```python
from build123d import *
from build123d import SkipClean  # not in build123d's __all__

# Parameters (mm, degrees)
F0_R      = 7.925
F1_DEPTH  = 9.6
F2_R      = 6.425
F3_DEPTH  = 2.5
F4_R      = 2.3
F4_R_2    = 1.575
F5_DEPTH  = 1.82
F12_W     = 4
F12_H     = 4.34
F13_DEPTH = 22.4162849636
F10_W     = 4
F10_H     = 4.34
F14_DEPTH = 22.4162849636
F17_DEPTH = 9.6
F15_R     = 2.4
F18_DEPTH = 15.851


with BuildPart() as f1:
    # F0 (on Top) → F1 (new body)
    with BuildSketch(Plane.XY):
        Circle(F0_R)
    extrude(amount=F1_DEPTH)

    # F2 (on face) → F3 (cut)
    with BuildSketch(Plane(origin=(0, 0, 0), x_dir=(1, 0, 0), z_dir=(0, 0, -1))):
        Circle(F2_R)
    extrude(amount=-F3_DEPTH, mode=Mode.SUBTRACT)

    # F4 (on face) → F5 (join)
    with BuildSketch(Plane.XY.offset(9.6)):
        with Locations((-4.1473636204, -3.8)):
            Circle(F4_R)
        with Locations((-4.1473636204, -3.8)):
            Circle(F4_R_2, mode=Mode.SUBTRACT)
        with Locations((-4.1473636204, 3.8)):
            Circle(F4_R)
        with Locations((-4.1473636204, 3.8)):
            Circle(F4_R_2, mode=Mode.SUBTRACT)
        with Locations((4.1473636204, 3.8)):
            Circle(F4_R)
        with Locations((4.1473636204, 3.8)):
            Circle(F4_R_2, mode=Mode.SUBTRACT)
        with Locations((4.1473636204, -3.8)):
            Circle(F4_R)
        with Locations((4.1473636204, -3.8)):
            Circle(F4_R_2, mode=Mode.SUBTRACT)
    extrude(amount=F5_DEPTH)

    # F12 (on face) → F13 (cut, through all)
    with BuildSketch(Plane(origin=(7.925, 7.925, 0), x_dir=(-0.7071067812, 0.7071067812, 0), z_dir=(0.7071067812, 0.7071067812, 0))):
        Rectangle(F12_W, F12_H)
    extrude(amount=-F13_DEPTH, mode=Mode.SUBTRACT)

    # F10 (on face) → F14 (cut, through all)
    with BuildSketch(Plane(origin=(7.925, -7.925, 0), x_dir=(0.7071067812, 0.7071067812, 0), z_dir=(0.7071067812, -0.7071067812, 0))):
        Rectangle(F10_W, F10_H)
    extrude(amount=-F14_DEPTH, mode=Mode.SUBTRACT)

    # F16 (on face) → F17 (join)
    with BuildSketch(Plane.XY.offset(9.6)):
        with BuildLine():
            Line((1.6, 2.828869032), (1.6, 3.5))
            Line((1.6, 3.5), (-1.6, 3.5))
            Line((-1.6, 3.5), (-1.6, 2.828869032))
            ThreePointArc((-1.6, 2.828869032), (-1.4275666191, 2.9196838096), (-1.25, 3))
            ThreePointArc((-1.25, 3), (0, 3.25), (1.25, 3))
            ThreePointArc((1.25, 3), (1.4275666191, 2.9196838096), (1.6, 2.828869032))
        make_face()
        with BuildLine():
            ThreePointArc((3.25, 0), (2.8073564077, 1.6374522894), (1.6, 2.828869032))
            Line((1.6, 2.828869032), (1.6, 1.9209372712))
            ThreePointArc((1.6, 1.9209372712), (2.2638462845, 1.0606601718), (2.5, 0))
            ThreePointArc((2.5, 0), (2.2638462845, -1.0606601718), (1.6, -1.9209372712))
            Line((1.6, -1.9209372712), (1.6, -2.828869032))
            ThreePointArc((1.6, -2.828869032), (2.8073564077, -1.6374522894), (3.25, 0))
        make_face()
        with BuildLine():
            Line((1.6, 1.9209372712), (1.6, 2.828869032))
            ThreePointArc((1.6, 2.828869032), (1.4275666191, 2.9196838096), (1.25, 3))
            Line((1.25, 3), (1.25, 2.1650635095))
            ThreePointArc((1.25, 2.1650635095), (1.4302183068, 2.0504817958), (1.6, 1.9209372712))
        make_face()
        with BuildLine():
            ThreePointArc((-1.25, 3), (-1.4275666191, 2.9196838096), (-1.6, 2.828869032))
            Line((-1.6, 2.828869032), (-1.6, 1.9209372712))
            ThreePointArc((-1.6, 1.9209372712), (-1.4302183068, 2.0504817958), (-1.25, 2.1650635095))
            Line((-1.25, 2.1650635095), (-1.25, 3))
        make_face()
        with BuildLine():
            Line((-1.6, 1.9209372712), (-1.6, 2.828869032))
            ThreePointArc((-1.6, 2.828869032), (-3.25, 0), (-1.6, -2.828869032))
            Line((-1.6, -2.828869032), (-1.6, -1.9209372712))
            ThreePointArc((-1.6, -1.9209372712), (-2.5, 0), (-1.6, 1.9209372712))
        make_face()
        with BuildLine():
            ThreePointArc((-1.25, -3), (-1.4275666191, -2.9196838096), (-1.6, -2.828869032))
            Line((-1.6, -2.828869032), (-1.6, -3.5))
            Line((-1.6, -3.5), (1.6, -3.5))
            Line((1.6, -3.5), (1.6, -2.828869032))
            ThreePointArc((1.6, -2.828869032), (1.4275666191, -2.9196838096), (1.25, -3))
            ThreePointArc((1.25, -3), (0, -3.25), (-1.25, -3))
        make_face()
        with BuildLine():
            Line((-1.6, -1.9209372712), (-1.6, -2.828869032))
            ThreePointArc((-1.6, -2.828869032), (-1.4275666191, -2.9196838096), (-1.25, -3))
            Line((-1.25, -3), (-1.25, -2.1650635095))
            ThreePointArc((-1.25, -2.1650635095), (-1.4302183068, -2.0504817958), (-1.6, -1.9209372712))
        make_face()
        with BuildLine():
            Line((1.6, -2.828869032), (1.6, -1.9209372712))
            ThreePointArc((1.6, -1.9209372712), (1.4302183068, -2.0504817958), (1.25, -2.1650635095))
            Line((1.25, -2.1650635095), (1.25, -3))
            ThreePointArc((1.25, -3), (1.4275666191, -2.9196838096), (1.6, -2.828869032))
        make_face()
        with BuildLine():
            Line((-1.25, 3), (1.25, 3))
            ThreePointArc((1.25, 3), (0, 3.25), (-1.25, 3))
        make_face()
        with BuildLine():
            Line((1.25, -3), (-1.25, -3))
            ThreePointArc((-1.25, -3), (0, -3.25), (1.25, -3))
        make_face()
    with SkipClean():  # cleaning this boolean's faces spoils the solid; the shape is the same uncleaned
        extrude(amount=-F17_DEPTH)

    # F15 (on offset) → F18 (cut, through all)
    with BuildSketch(Plane.YZ.offset(7.925)):
        with Locations((0, 5.4)):
            Circle(F15_R)
    with SkipClean():  # cleaning this boolean's faces spoils the solid; the shape is the same uncleaned
        extrude(amount=-F18_DEPTH, mode=Mode.SUBTRACT)


solid = f1.part
```
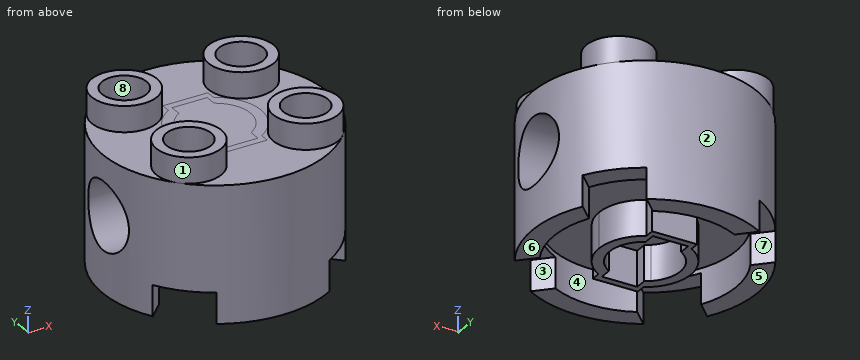
The listing builds one solid part. Answer for the finished solid, in the listing's coordinates (mm). Face numbers are marked on the shaded views. A direction names the side the tool comes from. Round coordinates to 2 decimals unless told otherwise and drop trailing zeros. Write each loop counter-clockwise with the first axis right and the second up, starting at its lowest first coordinate (ties: lowest second). Pieces come first, ordered by that corner, then holes. Notation, with made-up numbers: (14, -38.75) -> (57, -38.75) arc R21 cw to (57, -22.75) -> close; hole circle Ø1 at (-24.5, 21.25). An arc over 180 degrees is marked (long way). Write item = value, one per line.
1) Section B-B on y = 0.75 is taken. Write down the section's boundary in (x, z).
Check values:
outline = (-7.89, 0) -> (-6.38, 0) -> (-6.38, 2.5) -> (-3.16, 2.5) -> (-3.16, 0) -> (-2.38, 0) -> (-2.38, 2.5) -> (2.38, 2.5) -> (2.38, 0) -> (3.16, 0) -> (3.16, 2.5) -> (6.38, 2.5) -> (6.38, 0) -> (7.89, 0) -> (7.89, 3.12) -> (-7.89, 3.12) -> close; (-7.89, 7.68) -> (7.89, 7.68) -> (7.89, 9.6) -> (-7.89, 9.6) -> close
2) Straight lines are drawn through the part: line 1 along X through (y, z) = (-4.25, 10); line 2 along X through (y, z) = (-1.5, 0.5); line 3 along Z through (x, y) = (4, 0). For each, find the intervals that lie inside material, in ascending order. Write a range as [from, to].
Check values:
line_1 = [-6.4, -5.66], [-2.64, -1.89], [1.89, 2.64], [5.66, 6.4]
line_2 = [-7.78, -6.25], [-2.88, -2], [2, 2.88], [6.25, 7.78]
line_3 = [2.5, 3], [7.8, 9.6]
3) For a pull along Y with two mould halves and no side action, classify the marked faces 6, 7 and 8 as released by +Y, released by -Y, zero draft, split by the parting line, or undercut.
Check values:
face_6 = zero draft
face_7 = released by +Y
face_8 = undercut
4) Section D-D on y = 3.8 is taken. Write down the section's boundary in (x, z).
Check values:
outline = (-6.95, 0) -> (-6.63, 0) -> (-6.63, 2.17) -> (-5.18, 2.17) -> (-5.18, 2.5) -> (5.18, 2.5) -> (5.18, 2.17) -> (6.63, 2.17) -> (6.63, 0) -> (6.95, 0) -> (6.95, 9.6) -> (6.45, 9.6) -> (6.45, 11.42) -> (5.72, 11.42) -> (5.72, 9.6) -> (2.57, 9.6) -> (2.57, 11.42) -> (1.85, 11.42) -> (1.85, 9.6) -> (-1.85, 9.6) -> (-1.85, 11.42) -> (-2.57, 11.42) -> (-2.57, 9.6) -> (-5.72, 9.6) -> (-5.72, 11.42) -> (-6.45, 11.42) -> (-6.45, 9.6) -> (-6.95, 9.6) -> close
5) Section A-A on x = 0 is taken. Write down the section's boundary in (y, z) (3 decimals).
Check values:
outline = (-7.925, 0) -> (-6.425, 0) -> (-6.425, 2.5) -> (-3.5, 2.5) -> (-3.5, 0) -> (-3, 0) -> (-3, 2.5) -> (3, 2.5) -> (3, 0) -> (3.5, 0) -> (3.5, 2.5) -> (6.425, 2.5) -> (6.425, 0) -> (7.925, 0) -> (7.925, 9.6) -> (-7.925, 9.6) -> close; hole circle Ø4.8 at (0, 5.4)
6) Given pin 1 (0.7 mm diameter, centred on y = 3, z = 1, fed in from +X); pin 2 (4 mm diameter, centred on y = 5, z = 2, fed in from -X); pin 3 (0.9 mm diameter, centred on y = 2.5, z = 1.5, fed in from +X), each flat-ended and moving along its own axis, determine where each tip first touches the part or whether it passes through.
Check values:
pin_1 = 7.47
pin_2 = -7.34
pin_3 = 7.66
7) Section C-C on z = 7.25 is taken. Write down the section's boundary in (x, y) (3 decimals), plus the area to 3 significant figures.
Check values:
outline = (-7.776, -1.529) arc R7.925 ccw to (7.776, -1.529) -> close; (-7.776, 1.529) -> (7.776, 1.529) arc R7.925 ccw to start
area = 149 mm²
8) Which of the six approach directions +Z, -Z, +X, -X, +Y, -Y give full straight-line access (tool end or side, diameter ignored) to the marked faces 1, 2, 3, 4 and 5?
Check values:
face_1 = +Z
face_2 = +Z, -Z
face_3 = -Z, +X
face_4 = -Z
face_5 = -Z, +X, -X, +Y, -Y
